Here's how the part is built. I have some questions about the finished solid (model axes, mm). Face numbers are marked on the shaded views. Coordinates: 2 decimals unless noted, no trailing zeros. Write each loop counter-clockwise with the first axis right and the second up, starting at its lowest first coordinate (ties: lowest second). Pieces come first, ordered by that corner, then holes. Notation, with made-up numbers: (-17.5, 48.25) -> (22.5, 48.25) arc R24 ccw to (22.5, 85.25) -> close; hole circle Ø8 at (17, 48.25). An arc over 180 degrees is marked (long way). Put each result on its own line as item: value. Start each with the question number.
Item 1: If we mould it in two halves opening along X, with no side actions, what happens to the marked faces 1, 2 and 3? For each: released by +X, released by -X, zero draft, split by the parting line, or undercut.
Item 2: I want a section at B-B, the plane y = 3.5. List the corners of the cut face in (x, z) for me (1 decimal), then the cut area to 3 significant figures.
Item 3: I need wall thicknesses on line 1 (Z direction, x = -6, y = 4.5) (1 decimal); line 2 (X direction, y = -1.25, z = 2.5); line 3 (X direction, y = -1.5, z = 9). Which ranges of each line are inside material? Lowest first, please. Write a range as [from, to].
Item 4: I want a section at C-C, the plane z = 8. List the corners of the cut face in (x, y) for me (3 decimals), then the cut area to 3 significant figures.
Item 5: For pin 1 (1 mm diameter, centred on y = 1.5, z = 7, fed in from -X); pin 2 (4 mm diameter, centred on x = -0.5, y = 0.5, fed in from -Z); pin 3 (2 mm diameter, centred on x = 9.525, y = 3.175, fed in from -Z); pin 4 (2.5 mm diameter, centred on x = -9.525, y = 3.175, fed in from -Z) (3 decimals), each with a flat end and sliding along its axis, tell me the tip position at first contact or that it passes through.
Autodesk Inventor part; units mm, degrees
ref_plane "YZ Plane" through (0, 0, 0) normal (1, 0, 0) x (0, 1, 0)
ref_plane "XZ Plane" through (0, 0, 0) normal (0, 1, 0) x (-1, 0, 0)
ref_plane "XY Plane" through (0, 0, 0) normal (0, 0, 1) x (1, 0, 0)
sketch "Sketch1" plane through (0, 0, 0) normal (0, 0, 1) x (1, 0, 0)
  circle A0 centre (0, 0) radius 4.75
  dimension "d0" = 9.5
extrude "Extrusion1" add sketch "Sketch1" along normal blind 7.675
sketch "Sketch2" plane through (0, 0, 7.675) normal (0, 0, 1) x (1, 0, 0)
  circle A0 centre (0, 0) radius 4.75
  circle A1 centre (0, 0) radius 2.3813
  dimension "d3" = 4.7625
extrude "Extrusion2" cut sketch "Sketch2" against normal through all contours A1
sketch "Sketch3" plane through (0, 0, 7.675) normal (0, 0, 1) x (1, 0, 0)
  circle A0 centre (0, 0) radius 2.3813
  line L0 (-12.7, -6.35) -> (12.7, -6.35)
  line L1 (12.7, -6.35) -> (12.7, 6.35)
  line L2 (12.7, 6.35) -> (-12.7, 6.35)
  line L3 (-12.7, 6.35) -> (-12.7, -6.35)
  dimension "d6" = 25.4
  dimension "d7" = 12.7
extrude "Extrusion3" add sketch "Sketch3" along normal blind 1.5875
sketch "Sketch4" plane through (0, 0, 9.2625) normal (0, 0, 1) x (1, 0, 0)
  point P0 (-9.525, -3.175)
  point P1 (-9.525, 3.175)
  point P2 (9.525, 3.175)
  point P3 (9.525, -3.175)
hole "Hole1" at (-9.525, -3.175, 9.2625) at (-9.525, 3.175, 9.2625) at (9.525, 3.175, 9.2625) at (9.525, -3.175, 9.2625) direction (0, 0, -1) diameter 2.3876 end through all
properties part number "ferrous_insert"
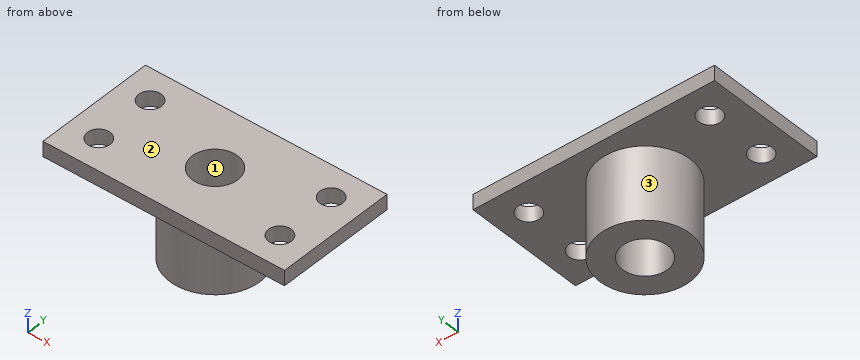
Calculated:
1. face 1: undercut
1. face 2: zero draft
1. face 3: split by the parting line
2. outline: (-12.7, 7.7) -> (-10.7, 7.7) -> (-10.7, 9.3) -> (-12.7, 9.3) -> close; (-8.4, 7.7) -> (-3.2, 7.7) -> (-3.2, 0) -> (3.2, 0) -> (3.2, 7.7) -> (8.4, 7.7) -> (8.4, 9.3) -> (-8.4, 9.3) -> close; (10.7, 7.7) -> (12.7, 7.7) -> (12.7, 9.3) -> (10.7, 9.3) -> close
2. area: 82.3 mm2
3. line 1: z = [7.7, 9.3]
3. line 2: x = [-4.58, -2.03], [2.03, 4.58]
3. line 3: x = [-12.7, -1.85], [1.85, 12.7]
4. outline: (-12.7, -6.35) -> (12.7, -6.35) -> (12.7, 6.35) -> (-12.7, 6.35) -> close; hole circle Ø2.388 at (-9.525, -3.175); hole circle Ø2.388 at (-9.525, 3.175); hole circle Ø4.763 at (0, 0); hole circle Ø2.388 at (9.525, -3.175); hole circle Ø2.388 at (9.525, 3.175)
4. area: 287 mm2
5. pin 1: stops at x = -4.64
5. pin 2: stops at z = 0
5. pin 3: passes through
5. pin 4: stops at z = 7.675
